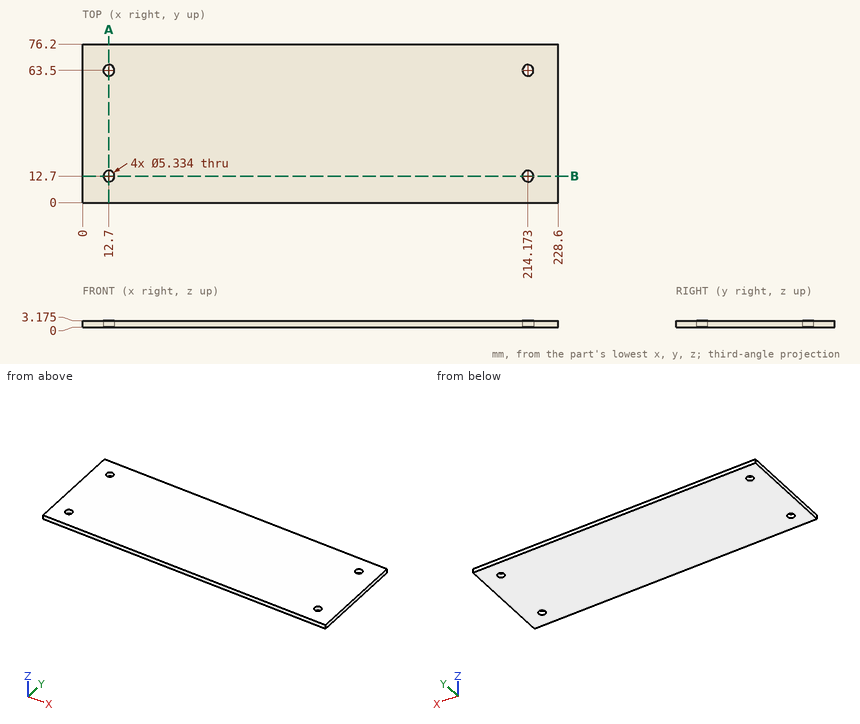
Geometry: see drawing. Coordinates: mm, zero at the bounding-box minimum. Give positions to 0.01 mm unless a question says otherwise; leave off trailing zeros. Loops run counter-clockwise (first coordinate to the right, second up) from the corner with the lowest first, then second, coordinate; pieces in that order, holes last. Notation, with made-up numbers: (2, 30) - (12, 30) arc R18 cw to (12, 35) - close; hole circle Ø8 at (-7, 82.5). An arc over 180 degrees is marked (long way). Answer as CSV lines item,"result". Start each with the question number.
1. Section A-A, the plane x = 12.7. Return loops of the section in (y, z) (1 decimal), plus the area to 3 significant figures.
2. Section B-B, the plane y = 12.7. Return loops of the section in (x, z) (1 decimal).
3. Pin query (flat end, axial travel): P1, Ø4.5, axis at x = 12.7, y = 12.7, coming from the -Z side. Return the tip coordinate at first contact, or that it passes through.
4. Ray query, L1, parallel to Y at x = 12.7, z = 2.5. Return the intervals inside material, ascending.
Answers:
1,outline,"(0, 0) - (10, 0) - (10, 3.2) - (0, 3.2) - close; (15.4, 0) - (60.8, 0) - (60.8, 3.2) - (15.4, 3.2) - close; (66.2, 0) - (76.2, 0) - (76.2, 3.2) - (66.2, 3.2) - close"
1,area,"208 mm2"
2,outline,"(0, 0) - (10, 0) - (10, 3.2) - (0, 3.2) - close; (15.4, 0) - (211.5, 0) - (211.5, 3.2) - (15.4, 3.2) - close; (216.8, 0) - (228.6, 0) - (228.6, 3.2) - (216.8, 3.2) - close"
3,P1,"passes through"
4,L1,"y = 0 to 10.03, 15.37 to 60.83, 66.17 to 76.2"
